Verification items for the finished model (mm, model axes). Round coordinates to 2 decimals unless told otherwise and drop trailing zeros. Write each loop counter-clockwise with the first axis right and the second up, starting at its lowest first coordinate (ties: lowest second). Pieces come first, ordered by that corner, then holes. Notation, with made-up numbers: (30.5, 45) -> (56.5, 45) arc R34 cw to (56.5, 79) -> close; hole circle Ø2 at (-15, 78.25). An arc over 180 degrees is marked (long way). Use CSV: the item, a comma, the result in double quotes.
```python
from build123d import *

# Parameters (mm, degrees)
SKETCH1_W           = 75
SKETCH1_H           = 25.4
SKETCH1_R           = 4.7625
SKETCH1_R_2         = 1.5
SKETCH1_R_3         = 4.5
BOSS_EXTRUDE1_DEPTH = 3.175
SKETCH2_R           = 1.984375
CUT_EXTRUDE1_DEPTH  = 3.175


with BuildPart() as part:
    # Sketch1 → Boss-Extrude1 (new body)
    with BuildSketch(Plane(origin=(0, 0, 0), x_dir=(1, 0, 0), z_dir=(0, 1, 0))):
        with Locations((37.5, 12.7)):
            Rectangle(SKETCH1_W, SKETCH1_H)
        with Locations(Location((43.7, 12.7, 0), (0, 0, 270))):
            Circle(SKETCH1_R, mode=Mode.SUBTRACT)
        with Locations(Location((6.35, 20.6375, 0), (0, 0, 270))):
            Circle(SKETCH1_R_2, mode=Mode.SUBTRACT)
        with Locations(Location((6.35, 4.7625, 0), (0, 0, 270))):
            Circle(SKETCH1_R_2, mode=Mode.SUBTRACT)
        with Locations(Location((6.35, 12.7, 0), (0, 0, 270))):
            Circle(SKETCH1_R_3, mode=Mode.SUBTRACT)
    extrude(amount=BOSS_EXTRUDE1_DEPTH)

    # Sketch2 → Cut-Extrude1 (cut)
    with BuildSketch(Plane(origin=(0, 0, 0), x_dir=(-1, 0, 0), z_dir=(0, -1, 0))):
        with Locations(Location((-18.3, 12.7, 0), (0, 0, 90))):
            Circle(SKETCH2_R)
        with Locations(Location((-69.1, 12.7, 0), (0, 0, 90))):
            Circle(SKETCH2_R)
    extrude(amount=-CUT_EXTRUDE1_DEPTH, mode=Mode.SUBTRACT)


solid = part.part
```
Q1. Section check A-A (x = 69.1). Record the cut outline in (y, z) (3 decimals), plus the area to 3 significant figures.
Filled in:
outline,"(0, -25.4) -> (3.175, -25.4) -> (3.175, -14.684) -> (0, -14.684) -> close; (0, -10.716) -> (3.175, -10.716) -> (3.175, 0) -> (0, 0) -> close"
area,"68.0 mm²"
Q2. Go/stop test with a flat-tipped pin: P1, Ø2.5, axis at x = 18.3, z = -12.7, coming from the -Y side. Record where the tip stops, or that it passes through.
Filled in:
P1,"through"
Q3. Material ranges on L1, parallel to X at y = 1.7, z = -12.7; L2, parallel to X at y = 2.3, z = -9; L3, parallel to Z at x = 5, y = 0.7, recorded low to high.
Filled in:
L1,"0 to 1.85, 10.85 to 16.32, 20.28 to 38.94, 48.46 to 67.12, 71.08 to 75"
L2,"0 to 3.79, 8.91 to 40.7, 46.7 to 75"
L3,"-25.4 to -21.29, -19.98 to -16.99, -8.41 to -5.42, -4.11 to 0"
Q4. Mould release check, pull along X, two halves, no side actions. Record for faces 1 (the flat face through (0, 2, -13)), 2 (the cylindrical face through (67.893, 1.565, -11.125)), 3 (the flat face through (37, 3.175, -13)): released by +X, released by -X, zero draft, split by the parting line, or undercut.
Filled in:
face 1,"released by -X"
face 2,"undercut"
face 3,"zero draft"
Q5. Section check B-B (y = 2.45). State how many separate pieces and enclosed holes the cut face has, plus the area to 3 significant figures.
Filled in:
separate pieces,"1"
enclosed holes,"6"
area,"1,730 mm²"
Q6. Section check D-D (x = 6.35). Record the cut outline in (y, z) (1 decimal).
Filled in:
outline,"(0, -25.4) -> (3.2, -25.4) -> (3.2, -22.1) -> (0, -22.1) -> close; (0, -19.1) -> (3.2, -19.1) -> (3.2, -17.2) -> (0, -17.2) -> close; (0, -8.2) -> (3.2, -8.2) -> (3.2, -6.3) -> (0, -6.3) -> close; (0, -3.3) -> (3.2, -3.3) -> (3.2, 0) -> (0, 0) -> close"
